Drawing for the job (mm, zero at the part's lowest x, y, z). Coordinates: 2 decimals unless noted, no trailing zeros. Loops run counter-clockwise (first coordinate to the right, second up) from the corner with the lowest first, then second, coordinate; pieces in that order, holes last. Notation, with made-up numbers: (84.25, 37) - (105.25, 37) arc R21 cw to (105.25, 45) - close; hole circle Ø10 at (61, 82.25). An arc over 180 degrees is marked (long way). Put each result on its own line as item: value.
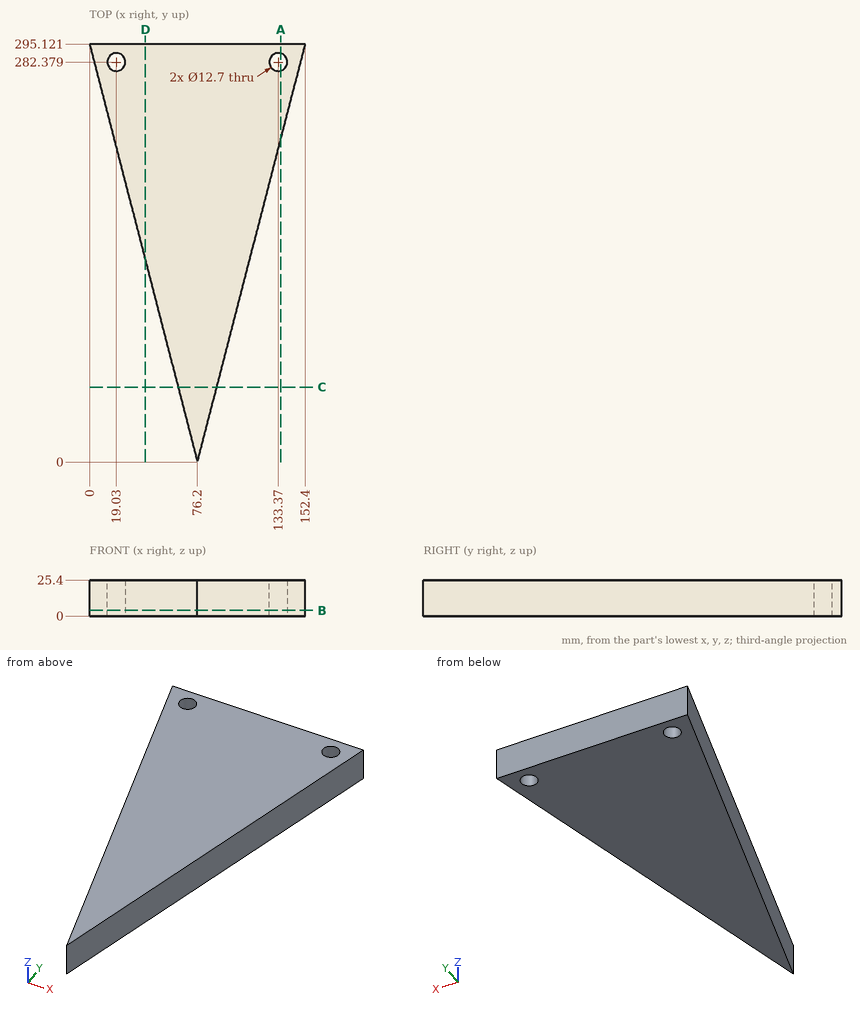
Q1. Slice it at D-D, the plane x = 39.5. Give the cut face in (y, z).
Determined:
outline: (142.14, 0) - (295.12, 0) - (295.12, 25.4) - (142.14, 25.4) - close
Q2. Slice it at C-C, the plane y = 53. Give the cut face in (x, z) (1 decimal), then the cut area to 3 significant figures.
Determined:
outline: (62.5, 0) - (89.9, 0) - (89.9, 25.4) - (62.5, 25.4) - close
area: 695 mm2
Q3. Wall check: L1, parallel to X at y = 282, z = 22.75; L2, parallel to X at y = 50.5, z = 16; L3, parallel to X at y = 237, z = 14. Give the ranges that are in metal, low to high. Write a range as from..to.
Determined:
L1: 3.39..12.69, 25.37..127.03, 139.71..149.01
L2: 63.16..89.24
L3: 15.01..137.39
Q4. Slice it at A-A, the plane x = 135. Give the cut face in (y, z), then the cut area to 3 significant figures.
Determined:
outline: (227.73, 0) - (276.24, 0) - (276.24, 25.4) - (227.73, 25.4) - close; (288.52, 0) - (295.12, 0) - (295.12, 25.4) - (288.52, 25.4) - close
area: 1,400 mm2
Q5. Slice it at B-B, the plane z = 4. Give the cut face in (x, y).
Determined:
outline: (0, 295.12) - (76.2, 0) - (152.4, 295.12) - close; hole circle Ø12.7 at (19.03, 282.38); hole circle Ø12.7 at (133.37, 282.38)
Q6. Pin check, flat tips, straight feed: pin 1 Ø3 at (y, z) = (231.5, 21) entering from -X; pin 2 Ø8 at (y, z) = (242, 15.5) entering from -X; pin 3 Ø2 at (y, z) = (237, 15) entering from -X. Stop position of each tip, or through.
Determined:
pin 1: x = 16.04
pin 2: x = 12.68
pin 3: x = 14.75
